Check sheet for the modelled part. Datum: model origin and axes. Units: mm. A direction names the side the tool comes from. Round coordinates to 2 decimals unless told otherwise and drop trailing zeros. Loops run counter-clockwise (first coordinate to the right, second up) from the corner with the lowest first, then second, coordinate; pieces in that order, holes last. Notation, with made-up numbers: M -2,5.25 L 37,5.25 A27 ccw 37,35.25 Z; hole C -2,89 d9. An arc over 180 degrees is marked long. Write item = value, one per line. Start each with the question number.
(1) Go/stop test with flat-tipped pins: P1, Ø5, axis at x = 21.46, z = 0, coming from the +Y side; P2, Ø9, axis at x = 2, z = 0, coming from the +Y side; P3, Ø1.4, axis at y = -14.5, z = 0, coming from the +X side. Record where each tip stops, or that it passes through.
(2) Cross-section at A-A on y = -19. Record the boundary of the cut face in (x, z), plus the area to 3 significant figures.
(3) Mould release check, pull along Y, two halves, no side actions. Record for faces 1 (the face through (-8.06, 20.04, -2.15)), 2 (the face through (17, 6, 0)), 3 (the face through (7, -17, 9)), 4 (the face through (-5.735, 9.512, 0.126)): pulls with the +Y half, pulls with the -Y half, needs draft (parallel to the pull), parting line crosses it, or undercut.
(4) Set-up check for faces 5 (the face through (20, 0, -2)), 6 (the face through (3, -54, -3)), 7 (the face through (-5.536, -26, 0)): record each of +Z, -Z, +X, -X, +Y, -Y from which the full face is reachable in a straight line by a thin tool's end or side.
(5) Cross-section at C-C on x = 10.5. Record the boundary of the cut face in (y, z).
(6) Cross-section at B-B on z = 0. Record the boundary of the cut face in (x, y).
(7) Scan lines: L1, parallel to X at y = 1.65, z = 0; L2, parallel to X at y = -55.4, z = 0; L3, parallel to X at y = -2.5, z = 1. Record each from-to range of solid material in increasing order. Write a range as from..to.
from build123d import *

# Parameters (mm, degrees)
BOSS_EXTRUDE1_DEPTH = 9
SKETCH2_R           = 2.15
CUT_EXTRUDE1_DEPTH  = 39.159314511
SKETCH3_R           = 2.15
CUT_EXTRUDE2_DEPTH  = 37.346022079
BOSS_EXTRUDE2_DEPTH = 18
CHAMFER1_SIZE       = 4
CHAMFER2_SIZE       = 2
FILLET1_R           = 6
CUT_EXTRUDE3_DEPTH  = 69.109715592
CUT_EXTRUDE4_DEPTH  = 73.836345899
SKETCH7_R           = 2.65
CUT_EXTRUDE5_DEPTH  = 94.724769777
CUT_EXTRUDE6_START  = -6
CUT_EXTRUDE6_DEPTH  = 88.724769777
CUT_EXTRUDE7_DEPTH  = 94.724769777


with BuildPart() as part:
    # Sketch1 → Boss-Extrude1 (new, symmetric)
    with BuildSketch(Plane.XY):
        Polygon((-14.732050808, 25.516660498), (0, 0), (29.464101615, 0), (29.464101615, 6), (3.464101615, 6), (-9.535898385, 28.516660498), align=None)
    extrude(amount=BOSS_EXTRUDE1_DEPTH, both=True)

    # Sketch2 → Cut-Extrude1 (cut, through all)
    with BuildSketch(Plane(origin=(0, 6, 0), x_dir=(1, 0, 0), z_dir=(0, 1, 0))):
        with Locations(Location((21.464101615, 0, 0), (0, 0, 270))):
            Circle(SKETCH2_R)
    extrude(amount=-CUT_EXTRUDE1_DEPTH, mode=Mode.SUBTRACT)

    # Sketch3 → Cut-Extrude2 (cut, through all)
    with BuildSketch(Plane(origin=(5.196152423, 3, 0), x_dir=(0, 0, -1), z_dir=(0.8660254037844397, 0.499999999999998, 0))):
        with Locations(Location((0, 21.464101615, 0), (0, 0, 90))):
            Circle(SKETCH3_R)
    extrude(amount=-CUT_EXTRUDE2_DEPTH, mode=Mode.SUBTRACT)

    # Sketch4 → Boss-Extrude2 (add)
    with BuildSketch(Plane(origin=(0, 0, -9), x_dir=(-1, 0, 0), z_dir=(0, 0, -1))):
        Polygon((0, 0), (-12.464101615, 0), (-12.464101615, -60), (5.535898385, -60), (5.535898385, 9.588457268), align=None)
    extrude(amount=-BOSS_EXTRUDE2_DEPTH)

    # Chamfer1
    chamfer1_edges = [part.edges().sort_by_distance(p)[0] for p in [
        (29.464101615, 3, 9),
        (-12.133974596, 27.016660498, 9),
        (29.464101615, 3, -9),
        (-12.133974596, 27.016660498, -9),
    ]]
    chamfer(chamfer1_edges, length=CHAMFER1_SIZE)

    # Chamfer2
    chamfer2_edges = [part.edges().sort_by_distance(p)[0] for p in [
        (12.464101615, 0, 0),
    ]]
    chamfer(chamfer2_edges, length=CHAMFER2_SIZE)

    # Fillet1
    fillet1_edges = [part.edges().sort_by_distance(p)[0] for p in [
        (-5.535898385, 9.588457268, 0),
    ]]
    fillet(fillet1_edges, radius=FILLET1_R)

    # Sketch5 → Cut-Extrude3 (cut, through all)
    with BuildSketch(Plane(origin=(5.196152423, 3, 0), x_dir=(0, 0, -1), z_dir=(0.8660254037844397, 0.4999999999999981, 0))):
        Polygon((-1.861954618, 22.539101615), (-2.482606158, 21.464101615), (-1.861954618, 20.389101615), align=None)
    extrude(amount=-CUT_EXTRUDE3_DEPTH, mode=Mode.SUBTRACT)

    # Sketch6 → Cut-Extrude4 (cut, through all)
    with BuildSketch(Plane(origin=(0, 6, 0), x_dir=(1, 0, 0), z_dir=(0, 1, 0))):
        Polygon((22.539101615, -1.861954618), (21.464101615, -2.482606158), (20.389101615, -1.861954618), align=None)
    extrude(amount=-CUT_EXTRUDE4_DEPTH, mode=Mode.SUBTRACT)

    # Sketch7 → Cut-Extrude5 (cut, through all)
    with BuildSketch(Plane.XZ.offset(60)):
        with Locations(Location((3.464101615, 0, 0), (0, 0, 270))):
            Circle(SKETCH7_R)
    extrude(amount=-CUT_EXTRUDE5_DEPTH, mode=Mode.SUBTRACT)

    # Sketch8 → Cut-Extrude6 (cut, through all)
    with BuildSketch(Plane.XZ.offset(60).offset(CUT_EXTRUDE6_START)):
        Polygon((3.464101615, 4.734272207), (-0.635898385, 2.367136104), (-0.635898385, -2.367136104), (3.464101615, -4.734272207), (7.564101615, -2.367136104), (7.564101615, 2.367136104), align=None)
    extrude(amount=-CUT_EXTRUDE6_DEPTH, mode=Mode.SUBTRACT)

    # Sketch10 → Cut-Extrude7 (cut, through all)
    with BuildSketch(Plane.XZ.offset(60)):
        Polygon((2.139101615, 2.29496732), (3.464101615, 3.059956427), (4.789101615, 2.29496732), align=None)
    extrude(amount=-CUT_EXTRUDE7_DEPTH, mode=Mode.SUBTRACT)


solid = part.part
Result:
q1.P1 = 6
q1.P2 = 16.33
q1.P3 = 12.46
q2.outline = M -5.54,-9 L 12.46,-9 L 12.46,9 L -5.54,9 Z; hole M -0.64,-2.37 L 3.46,-4.73 L 7.56,-2.37 L 7.56,2.37 L 3.46,4.73 L -0.64,2.37 Z
q2.area = 266 mm^2
q3.face_1 = undercut
q3.face_2 = pulls with the +Y half
q3.face_3 = needs draft
q3.face_4 = pulls with the -Y half
q4.face_5 = +Z, -Z, +X, -Y
q4.face_6 = +Y
q4.face_7 = +Z, -Z, -X, -Y
q5.outline = M -60,-9 L 6,-9 L 6,9 L -60,9 Z
q6.outline = M -14.73,25.52 L -11.81,20.45 L -6.61,23.45 L -9.54,28.52 Z; M -9.66,16.73 L -6.34,10.98 A6 cw -5.54,7.98 L -5.54,-60 L 0.81,-60 L 0.81,-54 L -0.64,-54 L -0.64,13.1 L -4.46,19.73 Z; M 6.11,-60 L 12.46,-60 L 12.46,-2 L 14.46,0 L 19.31,0 L 19.31,6 L 7.56,6 L 7.56,-54 L 6.11,-54 Z; M 23.61,0 L 29.46,0 L 29.46,6 L 23.61,6 Z
q7.L1 = -5.54..-0.64, 7.56..19.31, 23.61..29.46
q7.L2 = -5.54..0.81, 6.11..12.46
q7.L3 = -5.54..-0.64, 7.56..12.46
